```python
from build123d import *

# Parameters (mm, degrees)
SKETCH1_W             = 121.0056
SKETCH1_H             = 170.9928
BOSS_EXTRUDE1_DEPTH   = 3.048
BOSS_EXTRUDE1_TAPER   = 1
SKETCH2_W             = 120.899193924
SKETCH2_H             = 170.886393924
BOSS_EXTRUDE2_DEPTH   = 41.656
M3_TAPPED_HOLE1_D     = 2.5
M3_TAPPED_HOLE1_DEPTH = 4.7752
M3_TAPPED_HOLE1_TIP   = 0.751075774


with BuildPart() as part:
    # Sketch1 → Boss-Extrude1 (new body)
    with BuildSketch(Plane(origin=(0, 0, 0), x_dir=(1, 0, 0), z_dir=(0, 1, 0))):
        Rectangle(SKETCH1_W, SKETCH1_H)
    extrude(amount=BOSS_EXTRUDE1_DEPTH, taper=BOSS_EXTRUDE1_TAPER)

    # Sketch2 → Boss-Extrude2 (add)
    with BuildSketch(Plane(origin=(0, 3.048, 0), x_dir=(1, 0, 0), z_dir=(0, 1, 0))):
        Rectangle(SKETCH2_W, SKETCH2_H)
        Polygon((-55.852196962, 70.739), (-55.852196962, -70.739), (-38.9255, -70.739), (-38.9255, -80.845796962), (38.9255, -80.845796962), (38.9255, -70.739), (55.852196962, -70.739), (55.852196962, 70.739), (38.9255, 70.739), (38.9255, 80.845796962), (-38.9255, 80.845796962), (-38.9255, 70.739), align=None, mode=Mode.SUBTRACT)
    extrude(amount=BOSS_EXTRUDE2_DEPTH)

    # M3 Tapped Hole1
    with Locations(Plane(origin=(0, 3.048, 0), x_dir=(1, 0, 0), z_dir=(0, 1, 0))):
        with Locations((-45.466, 65.8876), (45.466, -65.8876), (45.466, 65.8876), (-45.466, -65.8876)):
            Hole(M3_TAPPED_HOLE1_D / 2, depth=M3_TAPPED_HOLE1_DEPTH)
            with Locations((0, 0, -(M3_TAPPED_HOLE1_DEPTH + M3_TAPPED_HOLE1_TIP / 2))):  # 118° drill point
                Cone(0, M3_TAPPED_HOLE1_D / 2, M3_TAPPED_HOLE1_TIP, mode=Mode.SUBTRACT)


solid = part.part
```
Design review of the part built by this model. Coordinates are the model's own, in mm. Give positions to 0.01 mm unless a question says otherwise; leave off trailing zeros. Order: outer loops, then holes, each group sorted by start corner. A loop starts at its lowest first (then second) coordinate and runs counter-clockwise, first axis right, second up. Notation, with made-up numbers: (59.25, 43.25) -> (106.25, 43.25) arc R25 cw to (106.25, 73.25) -> close; hole circle Ø9 at (-28, 56). An arc over 180 degrees is marked (long way). Write item = value, one per line. Start each with the question number.
(1) To check wall thickness, follow line 1 along Z through (x, y) = (19, 41.5); line 2 along X through (y, z) = (21, 48); line 3 along Z through (x, y) = (-44, 37.5). State the ranges of each line that lie inside material, in increasing order.
(2) We need section A-A on y = 24.5. Write out the cut boundary in (x, z), plus the area to 3 significant figures.
(3) Mouldability with a two-part tool opening along Z and no side actions: class faces 1 (the face through (-1, 24, 85.443)), 2 (the face through (-47, 24, -70.739)), 3 (the face through (-58, 44.704, -7)) as +Z half, -Z half, draft (parallel to the pull), parting line (faces both ways), or undercut.
(4) For pin 1 (8 mm diameter, centred on y = 38, z = 40.5, fed in from -X); pin 2 (8.5 mm diameter, centred on x = 45.5, y = 28, fed in from +Z); pin 3 (8 mm diameter, centred on y = 22.5, z = 74.5, fed in from +X), all flat-tipped, find the tip position at first contact; note any pin that passes through.
Numbers:
q1.line_1 = -85.44 to -80.85, 80.85 to 85.44
q1.line_2 = -60.45 to -55.85, 55.85 to 60.45
q1.line_3 = -85.44 to -70.74, 70.74 to 85.44
q2.outline = (-60.45, -85.44) -> (60.45, -85.44) -> (60.45, 85.44) -> (-60.45, 85.44) -> close; hole (-55.85, -70.74) -> (-38.93, -70.74) -> (-38.93, -80.85) -> (38.93, -80.85) -> (38.93, -70.74) -> (55.85, -70.74) -> (55.85, 70.74) -> (38.93, 70.74) -> (38.93, 80.85) -> (-38.93, 80.85) -> (-38.93, 70.74) -> (-55.85, 70.74) -> close
q2.area = 3,280 mm^2
q3.face_1 = +Z half
q3.face_2 = undercut
q3.face_3 = draft
q4.pin_1 = -60.45
q4.pin_2 = 85.44
q4.pin_3 = 60.45
